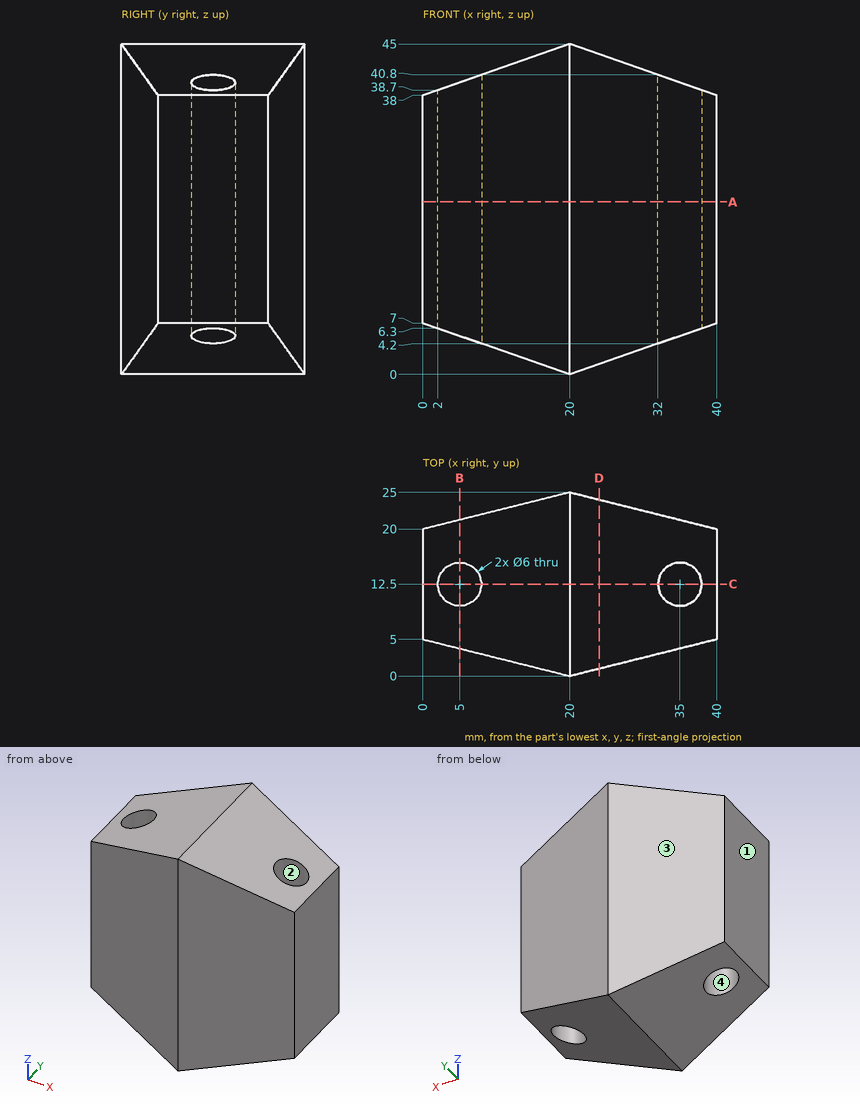
Check sheet for the drawn part. Datum: minimum x, y, z corner. Units: mm. Give positions to 0.01 mm unless a question says otherwise; leave off trailing zeros. Write each loop counter-clockwise with the first axis right and the second up, starting at its lowest first coordinate (ties: lowest second). Pieces come first, ordered by that corner, then holes. Notation, with made-up numbers: M 42,74 L 97,74 A10 ccw 97,87 Z; hole C 48.5,3.25 d11. An arc over 180 degrees is marked long. One line per question, with ' | ' between items.
1) Gauge pin test, flat ends, axial feed: pin 1 Ø2 at (x, z) = (15.5, 13.5) entering from -Y (3 decimals); pin 2 Ø6 at (x, z) = (29.5, 39) entering from -Y (3 decimals); pin 3 Ø8 at (y, z) = (9, 15) entering from -X; pin 4 Ø4 at (x, y) = (17, 18) entering from +Z. Record the tip position at first contact, or that the pin passes through.
Result:
pin 1: stops at y = 0.875 | pin 2: stops at y = 1.625 | pin 3: stops at x = 0 | pin 4: stops at z = 44.65
2) Thickness scan on line 1 along X through (y, z) = (14.5, 31); line 2 along Y through (x, z) = (5, 29). Record the ranges inside material, lowest first. Write a range as [from, to].
Result:
line 1: x = [0, 2.76], [7.24, 32.76], [37.24, 40] | line 2: y = [3.75, 9.5], [15.5, 21.25]
3) Section check A-A on z = 23.5. Enter the section's corners in (x, y).
Result:
outline: M 0,5 L 20,0 L 40,5 L 40,20 L 20,25 L 0,20 Z; hole C 5,12.5 d6; hole C 35,12.5 d6
4) Section check B-B on x = 5. Enter the section's corners in (y, z), plus the area to 3 significant figures.
Result:
outline: M 3.75,5.25 L 9.5,5.25 L 9.5,39.75 L 3.75,39.75 Z; M 15.5,5.25 L 21.25,5.25 L 21.25,39.75 L 15.5,39.75 Z | area: 397 mm2
5) Section check D-D on x = 24. Enter the section's corners in (y, z), plus the area to 3 significant figures.
Result:
outline: M 1,1.4 L 24,1.4 L 24,43.6 L 1,43.6 Z | area: 971 mm2
6) Section check C-C on y = 12.5. Enter the section's corners in (x, z).
Result:
outline: M 0,7 L 2,6.3 L 2,38.7 L 0,38 Z; M 8,4.2 L 20,0 L 32,4.2 L 32,40.8 L 20,45 L 8,40.8 Z; M 38,6.3 L 40,7 L 40,38 L 38,38.7 Z
7) Mould release check, pull along Y, two halves, no side actions. Record for the marked faces 1, 2, 3 and 4: released by +Y, released by -Y, zero draft, split by the parting line, or undercut.
Result:
face 1: zero draft | face 2: undercut | face 3: released by +Y | face 4: undercut
